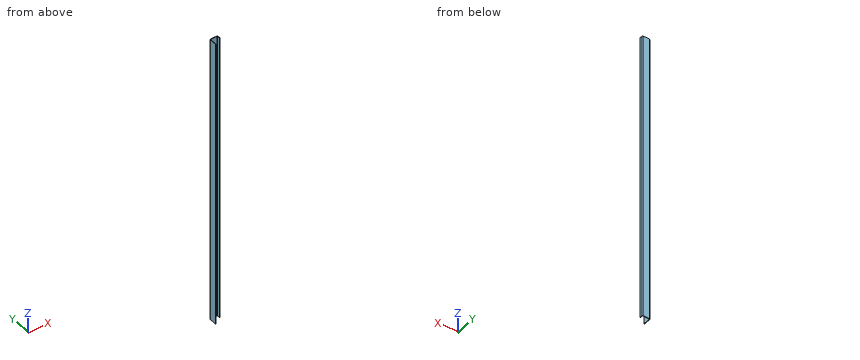
Autodesk Inventor part; units mm, degrees
ref_plane "YZ Plane" through (0, 0, 0) normal (1, 0, 0) x (0, 1, 0)
ref_plane "XZ Plane" through (0, 0, 0) normal (0, 1, 0) x (-1, 0, 0)
ref_plane "XY Plane" through (0, 0, 0) normal (0, 0, 1) x (1, 0, 0)
sketch "Sketch1" plane through (0, 0, 0) normal (0, 0, 1) x (1, 0, 0)
  line L0 (0, 0) -> (0, 25)
  line L1 (0, 25) -> (25, 25)
  line L2 (25, 25) -> (25, 15)
  dimension "d0" = 25
  dimension "d1" = 25
  dimension "d2" = 10
contour flange "Contour Flange1" sketch "Sketch1" thickness 1.5 bend radius 1.5 width 930 along (0, 0, 1) mid plane yes both sides no wall seen from (0, 12.5, 0) lies toward (1, 0, 0) curves L0 L1 L2
bend "Bend1"
corner "Corner1"
equation "\"d3\" = BendReliefWidth"
equation "\"d4\" = BendReliefDepth"
equation "\"d5\" = MinimumRemnant"
equation "\"d6\" = BendRadius"
equation "\"d8\" = BendRadius"
equation "\"d10\" = CornerReliefSize"
equation "\"d11\" = GapSize"
equation "\"d12\" = JacobiRadiusSize"
equation "\"BendRadius\" = Thickness"
equation "\"BendReliefWidth\" = Thickness"
equation "\"BendReliefDepth\" = 0.5 * Thickness"
equation "\"CornerReliefSize\" = 4 * Thickness"
equation "\"MinimumRemnant\" = 2 * Thickness"
equation "\"TransitionRadius\" = BendRadius"
equation "\"JacobiRadiusSize\" = BendRadius"
equation "\"GapSize\" = Thickness"
properties part number "Perfil \"J\"" material "Stainless Steel"
Work out the finished part from the listing and answer in its coordinate system (mm). Round coordinates to 2 decimals unless told otherwise and drop trailing zeros. Loops run counter-clockwise (first coordinate to the right, second up) from the corner with the lowest first, then second, coordinate; pieces in that order, holes last. Notation, with made-up numbers: M 23.25,7.5 L 74.25,7.5 A10 cw 74.25,13.5 Z; hole C 88.5,11 d8. An arc over 180 degrees is marked long. One line per question, with ' | ' between items. Start each with the question number.
(1) A cutting plane is placed at A-A on z = 101. Write down the section's boundary in (x, y).
(2) A cutting plane is placed at B-B on y = 10.5. Write down the section's boundary in (x, z), plus the area to 4 significant figures.
(3) Find the intervals of material crossed by line 1 (X direction, y = 21, z = -202); line 2 (Y direction, x = 2.75, z = -394); line 3 (X direction, y = 1.5, z = 276), in increasing order.
(4) A cutting plane is placed at C-C on x = 7. Write down the section's boundary in (y, z), plus the area to 4 significant figures.
(5) Flat-ended cylindrical pins translate along their axes: pin 1 Ø5.5 at (x, z) = (14, -223) entering from -Y; pin 2 Ø0.8 at (x, z) = (24.5, -139.5) entering from -Y. Find the tip coordinate at first contact, or state that the pin passes through.
Geometry check:
1) outline: M 0,0 L 1.5,0 L 1.5,22 A1.5 cw 3,23.5 L 22,23.5 A1.5 cw 23.5,22 L 23.5,15 L 25,15 L 25,22 A3 ccw 22,25 L 3,25 A3 ccw 0,22 Z
2) outline: M 0,-465 L 1.5,-465 L 1.5,465 L 0,465 Z | area: 1,395 mm²
3) line 1: x = 0 to 1.5, 23.5 to 25 | line 2: y = 23.48 to 24.99 | line 3: x = 0 to 1.5
4) outline: M 23.5,-465 L 25,-465 L 25,465 L 23.5,465 Z | area: 1,395 mm²
5) pin 1: stops at y = 23.5 | pin 2: stops at y = 15
